Source: three-view drawing plus pictorial views. Frame: mm from the lowest corner of the part. Round coordinates to 2 decimals unless told otherwise and drop trailing zeros. Loops run counter-clockwise (first coordinate to the right, second up) from the corner with the lowest first, then second, coordinate; pieces in that order, holes last. Notation, with made-up numbers: (-29, 84.25) -> (8, 84.25) arc R37 ccw to (8, 121.25) -> close; hole circle Ø3 at (68.5, 53.5). An arc over 180 degrees is marked (long way). One line per question, with ' | ' between items. Start each with the question number.
Q1. Material intervals for L1, parallel to Z at x = 14, y = 3.8; L2, parallel to X at y = 0.5, z = 2.75; L3, parallel to Z at x = 3.75, y = 2, sorted ascending.
Q2. Cut plane B-B on y = 0.9. Return loops of the section in (x, z).
Q3. Cut plane C-C on z = 3. Return loops of the section in (x, y).
Q4. Cut plane D-D on y = 4.75. Return loops of the section in (x, z), and give its area (3 significant figures).
Q5. Contact query for a flat-ended pin moving along its axis: P1, Ø2.5, axis at x = 3, z = 3, coming from the +Y side. Output: stop coordinate, or through.
Q6. Cut plane A-A on x = 3. Return loops of the section in (y, z), and give its area (3 significant figures).
Q7. Mould query, pull axis X, two halves, no side actions, for the marked faces 1, 2 and 3. Classes: pulls with the +X half, pulls with the -X half, needs draft (parallel to the pull), parting line crosses it, or undercut.
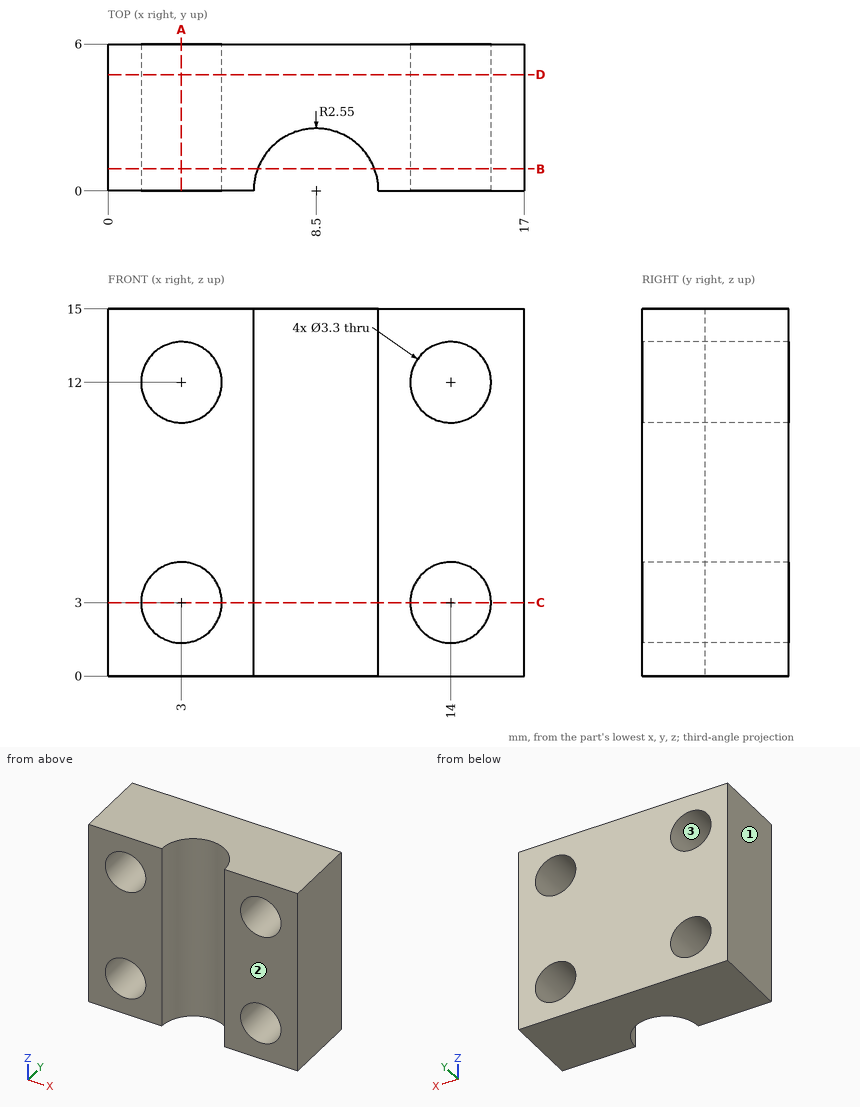
Results:
1) L1: 0 to 1.35, 4.65 to 10.35, 13.65 to 15 | L2: 0 to 1.37, 4.63 to 6, 11 to 12.37, 15.63 to 17 | L3: 0 to 1.53, 4.47 to 10.53, 13.47 to 15
2) outline: (0, 0) -> (6.11, 0) -> (6.11, 15) -> (0, 15) -> close; (10.89, 0) -> (17, 0) -> (17, 15) -> (10.89, 15) -> close; hole circle Ø3.3 at (3, 3); hole circle Ø3.3 at (3, 12); hole circle Ø3.3 at (14, 3); hole circle Ø3.3 at (14, 12)
3) outline: (0, 0) -> (1.35, 0) -> (1.35, 6) -> (0, 6) -> close; (4.65, 0) -> (5.95, 0) arc R2.55 cw to (11.05, 0) -> (12.35, 0) -> (12.35, 6) -> (4.65, 6) -> close; (15.65, 0) -> (17, 0) -> (17, 6) -> (15.65, 6) -> close
4) outline: (0, 0) -> (17, 0) -> (17, 15) -> (0, 15) -> close; hole circle Ø3.3 at (3, 3); hole circle Ø3.3 at (3, 12); hole circle Ø3.3 at (14, 3); hole circle Ø3.3 at (14, 12) | area: 221 mm^2
5) P1: through
6) outline: (0, 0) -> (6, 0) -> (6, 1.35) -> (0, 1.35) -> close; (0, 4.65) -> (6, 4.65) -> (6, 10.35) -> (0, 10.35) -> close; (0, 13.65) -> (6, 13.65) -> (6, 15) -> (0, 15) -> close | area: 50.4 mm^2
7) face 1: pulls with the -X half | face 2: needs draft | face 3: undercut
